Can you work these out from the drawing? Everything is in mm from the part's minimum corner. Coordinates: 2 decimals unless noted, no trailing zeros. Loops run counter-clockwise (first coordinate to the right, second up) from the corner with the lowest first, then second, coordinate; pieces in that order, holes last. Notation, with made-up numbers: (-36, 8) -> (-25, 8) arc R20 cw to (-25, 40) -> close; hole circle Ø1 at (40, -35). An arc over 180 degrees is marked (long way). One line per question, with ' | ' between items.
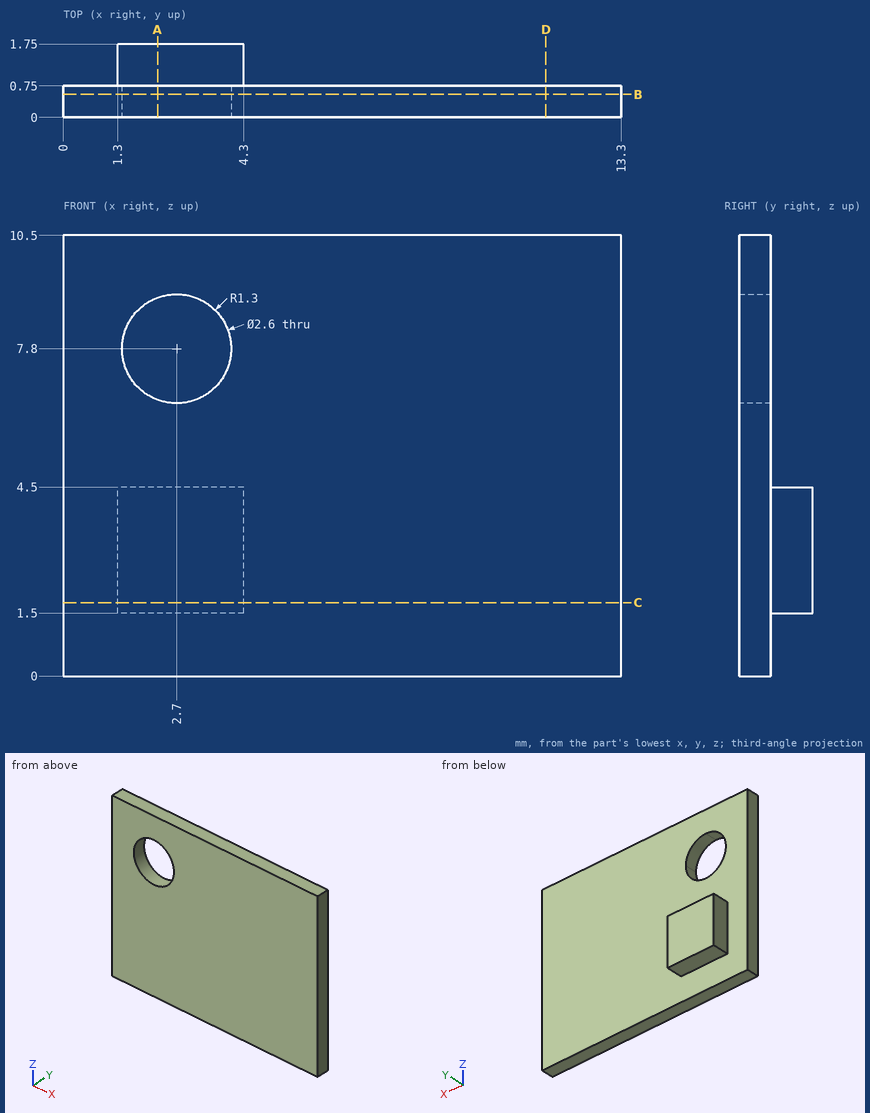
Q1. For pin 1 (2.5 mm diameter, centred on x = 2.7, z = 7.8, fed in from +Y); pin 2 (1 mm diameter, centred on x = 5, z = 6, fed in from +Y); pin 3 (1 mm diameter, centred on y = 1.5, z = 3, fed in from -X); pin 4 (0.8 mm diameter, centred on y = 1.5, z = 3.5, fed in from +X), each with a flat end and sliding along its axis, tell me the tip position at first contact or that it passes through.
Values follow:
pin 1: passes through | pin 2: stops at y = 0.75 | pin 3: stops at x = 1.3 | pin 4: stops at x = 4.3
Q2. Imagine slicing it at A-A on x = 2.25. Write out the boundary of the cut face in (y, z), plus the area to 3 significant figures.
Values follow:
outline: (0, 0) -> (0.75, 0) -> (0.75, 1.5) -> (1.75, 1.5) -> (1.75, 4.5) -> (0.75, 4.5) -> (0.75, 6.58) -> (0, 6.58) -> close; (0, 9.02) -> (0.75, 9.02) -> (0.75, 10.5) -> (0, 10.5) -> close | area: 9.05 mm2
Q3. Imagine slicing it at B-B on y = 0.55. Write out the boundary of the cut face in (x, z).
Values follow:
outline: (0, 0) -> (13.3, 0) -> (13.3, 10.5) -> (0, 10.5) -> close; hole circle Ø2.6 at (2.7, 7.8)
Q4. Imagine slicing it at C-C on z = 1.75. Write out the boundary of the cut face in (x, y).
Values follow:
outline: (0, 0) -> (13.3, 0) -> (13.3, 0.75) -> (4.3, 0.75) -> (4.3, 1.75) -> (1.3, 1.75) -> (1.3, 0.75) -> (0, 0.75) -> close
Q5. Imagine slicing it at D-D on x = 11.5. Write out the boundary of the cut face in (y, z), plus the area to 4 significant figures.
Values follow:
outline: (0, 0) -> (0.75, 0) -> (0.75, 10.5) -> (0, 10.5) -> close | area: 7.875 mm2
Q6. Please list where these lines run through material, in increasing order: L1, parallel to Z at x = 2.7, y = 0.5; L2, parallel to X at y = 0.25, z = 7.8; L3, parallel to Y at x = 12, z = 2. Write a range as [from, to].
Values follow:
L1: z = [0, 6.5], [9.1, 10.5] | L2: x = [0, 1.4], [4, 13.3] | L3: y = [0, 0.75]
